CAD build for the part. Positions are in the model's coordinates, mm. A direction names the side the tool comes from. Coordinates: 2 decimals unless noted, no trailing zeros. Write each loop counter-clockwise with the first axis right and the second up, starting at its lowest first coordinate (ties: lowest second). Pieces come first, ordered by that corner, then holes.
```python
from build123d import *

# Parameters (mm, degrees)
SKETCH153_W             = 7
SKETCH153_H             = 17
PAD051_DEPTH            = 20
SKETCH152_R             = 1.5
POCKET087_DEPTH         = 20
POCKET161_DEPTH         = 10
CHAMFER042_1_SIZE2      = 8
CHAMFER042_1_SIZE       = 2
CHAMFER042_2_SIZE2      = 8
CHAMFER042_2_SIZE       = 2
SKETCH276_W             = 3
SKETCH276_H             = 3
POCKET164_DEPTH         = 2
CHAMFER_SIZE            = 0.4
BODY018_PLACEMENT_ANGLE = 180


with BuildPart() as innerplateend:
    # Sketch153 → Pad051 (new body, symmetric)
    with BuildSketch(Plane.XZ):
        with Locations((39.5, -1.5)):
            Rectangle(SKETCH153_W, SKETCH153_H)
    extrude(amount=PAD051_DEPTH, both=True)

    # Sketch152 → Pocket087 (cut, symmetric)
    with BuildSketch(Plane.XZ):
        with Locations((40, -1)):
            Circle(SKETCH152_R)
    extrude(amount=POCKET087_DEPTH, both=True, mode=Mode.SUBTRACT)

    # Sketch250 → Revolution004 (revolve)
    with BuildSketch(Plane.XZ):
        Polygon((52, 0), (43, 0), (43, 5), (44, 5), (45, 4), (52, 4), align=None)
    revolve(axis=Axis((0, 0, 0), (1, 0, 0)))

    # Sketch267 → Pocket161 (cut)
    with BuildSketch(Plane.XZ.offset(12)):
        Polygon((43, -7.5), (36, -7.499985956), (36, 3), (43, 3), align=None)
    pocket161 = extrude(amount=POCKET161_DEPTH, mode=Mode.SUBTRACT)

    # Mirrored: Pocket161 across XZ
    add(pocket161.mirror(Plane.XZ), mode=Mode.SUBTRACT)

    # Chamfer042 1
    chamfer042_1_edges = [innerplateend.edges().sort_by_distance(p)[0] for p in [
        (39.5, 20, 7),
    ]]
    chamfer042_1_side = innerplateend.faces().sort_by_distance((39.5, 20, 5))[0]
    chamfer(chamfer042_1_edges, length=CHAMFER042_1_SIZE, length2=CHAMFER042_1_SIZE2, reference=chamfer042_1_side)

    # Chamfer042 2
    chamfer042_2_edges = [innerplateend.edges().sort_by_distance(p)[0] for p in [
        (39.5, -20, 7),
    ]]
    chamfer042_2_side = innerplateend.faces().sort_by_distance((39.5, -20, 5))[0]
    chamfer(chamfer042_2_edges, length=CHAMFER042_2_SIZE, length2=CHAMFER042_2_SIZE2, reference=chamfer042_2_side)

    # Sketch276 (on Face21 of Chamfer042) → Pocket164 (cut)
    with BuildSketch(Plane(origin=(52, 0, 0), x_dir=(0, 0, 1), z_dir=(1, 0, 0))):
        Rectangle(SKETCH276_W, SKETCH276_H)
    extrude(amount=-POCKET164_DEPTH, mode=Mode.SUBTRACT)

    # Chamfer
    chamfer_edges = [innerplateend.edges().sort_by_distance(p)[0] for p in [
        (52, 0, 1.5),
        (52, 1.5, 0),
        (52, 0, -1.5),
        (52, -1.5, 0),
    ]]
    chamfer(chamfer_edges, length=CHAMFER_SIZE)


with BuildPart() as innerplateend_1:
    # Body018 placement: moved
    add(innerplateend.part.rotate(Axis((0, 0, 0), (0, 0, 1)), BODY018_PLACEMENT_ANGLE))


with BuildPart() as ref_innerplateend:
    # Part__Mirroring002: instance of InnerPlateEnd
    add(innerplateend_1.part.mirror(Plane(origin=(0, 0, 0), x_dir=(0, -1, 0), z_dir=(1, 0, 0))))


solid = ref_innerplateend.part
```
Item 1: Which spindle directions (+Z, -Z, +X, -X, +Y, -Y) get a long thin tool onto all of the face, cutting with end or side? Do faces 1 (the flat face through (39, 16, 3)), 2 (the cylindrical face through (43.507, 4.216, 2.688)), 3 (the flat face through (39, -16, 3)), 4 (the flat face through (39, -20, -9)), 5 (the cylindrical face through (38.5, 0.17, -0.93)). Say none if no direction does.
Item 2: Two-plate mould, pull along Y, no slides. Class faces 6 (the cylindrical face through (48.549, 1.201, 3.815)), 7 (the flat face through (51, -1.5, 0)), 8 (the flat face through (39, 20, -9)), 9 (the flat face through (51, 0, 1.5)): +Y half, -Y half, draft (parallel to the pull), parting line (faces both ways), or undercut.
Item 3: Saw through at B-B, the plane y = 0. Write the cut outline in (x, z), and give its area (3 significant figures).
Item 4: Saw through at D-D, the plane z = 0. Write the cut outline in (x, y).
Item 5: Saw through at A-A, the plane x = 40. Write the cut outline in (y, z), and give its area (3 significant figures).
Item 6: Saw through at C-C, the plane x = 42.5. Write the cut outline in (y, z).
Item 7: Flat gauge pins, fed straight in: pin 1 Ø5.5 at (x, y) = (39, -16.5) entering from +Z; pin 2 Ø8 at (x, z) = (50, 4.5) entering from +Y; pin 3 Ø0.5 at (x, z) = (51, 0.5) entering from -Y. Where does each tip first touch, or does it go through?
Item 8: Wall check: line 1 along Z through (x, y) = (40, -4.5); line 2 along X through (y, z) = (4.5, -8); line 3 along Y through (x, z) = (37.25, 2.75). Give the ranges that are in metal, low to high.
Working result:
1. face 1: +X, -X, +Y
1. face 2: +X
1. face 3: +X, -X, -Y
1. face 4: +Z, -Z, +X, -X, -Y
1. face 5: +Y, -Y
2. face 6: parting line
2. face 7: undercut
2. face 8: +Y half
2. face 9: undercut
3. outline: (36, -10) - (43, -10) - (43, -5) - (44, -5) - (45, -4) - (52, -4) - (52, -1.9) - (51.6, -1.5) - (50, -1.5) - (50, 1.5) - (51.6, 1.5) - (52, 1.9) - (52, 4) - (45, 4) - (44, 5) - (43, 5) - (43, 7) - (36, 7) - close; hole circle Ø3 at (40, -1)
3. area: 181 mm2
4. outline: (36, -12) - (38.88, -12) - (38.88, 12) - (36, 12) - close; (41.12, -12) - (43, -12) - (43, -5) - (44, -5) - (45, -4) - (52, -4) - (52, -1.9) - (51.6, -1.5) - (50, -1.5) - (50, 1.5) - (51.6, 1.5) - (52, 1.9) - (52, 4) - (45, 4) - (44, 5) - (43, 5) - (43, 12) - (41.12, 12) - close
5. outline: (-20, -10) - (20, -10) - (20, -7.5) - (12, -7.5) - (12, -2.5) - (-12, -2.5) - (-12, -7.5) - (-20, -7.5) - close; (-20, 3) - (-12, 3) - (-12, 0.5) - (12, 0.5) - (12, 3) - (20, 3) - (20, 5) - (12, 7) - (-12, 7) - (-20, 5) - close
5. area: 424 mm2
6. outline: (-20, -10) - (20, -10) - (20, -7.5) - (12, -7.5) - (12, 3) - (20, 3) - (20, 5) - (12, 7) - (-12, 7) - (-20, 5) - (-20, 3) - (-12, 3) - (-12, -7.5) - (-20, -7.5) - close
7. pin 1: stops at z = 6.56
7. pin 2: stops at y = 3.97
7. pin 3: stops at y = -3.99
8. line 1: z = -10 to -2.5, 0.5 to 7
8. line 2: x = 36 to 43
8. line 3: y = -12 to 12
